Check sheet for the modelled part. Datum: model origin and axes. Units: mm. A direction names the side the tool comes from. Coordinates: 2 decimals unless noted, no trailing zeros. Loops run counter-clockwise (first coordinate to the right, second up) from the corner with the lowest first, then second, coordinate; pieces in that order, holes last. Notation, with made-up numbers: M -17,52.25 L 14,52.25 A19 ccw 14,58.25 Z; hole C -30,9 d7. An arc over 180 degrees is marked long. Answer as CSV lines item,"result". Start each with the question number.
from build123d import *

# Parameters (mm, degrees)
SKETCH052_W     = 15
SKETCH052_H     = 44
PAD029_DEPTH    = 1
SKETCH053_W     = 10.5
SKETCH053_H     = 39.5
PAD030_DEPTH    = 30.5
CHAMFER028_SIZE = 0.5
CHAMFER029_SIZE = 0.5


with BuildPart() as part:
    # Sketch052 → Pad029 (new body)
    with BuildSketch(Plane.XY):
        Rectangle(SKETCH052_W, SKETCH052_H)
    extrude(amount=-PAD029_DEPTH)

    # Sketch053 (on Face5 of Pad029) → Pad030 (join)
    with BuildSketch(Plane.XY):
        Rectangle(SKETCH053_W, SKETCH053_H)
    extrude(amount=PAD030_DEPTH)

    # Chamfer028
    chamfer028_edges = [part.edges().sort_by_distance(p)[0] for p in [
        (-5.25, -19.75, 15.25),
        (5.25, -19.75, 15.25),
        (0, -19.75, 30.5),
        (-5.25, 0, 30.5),
        (5.25, 0, 30.5),
        (5.25, 19.75, 15.25),
        (0, 19.75, 30.5),
        (-5.25, 19.75, 15.25),
    ]]
    chamfer(chamfer028_edges, length=CHAMFER028_SIZE)

    # Chamfer029
    chamfer029_edges = [part.edges().sort_by_distance(p)[0] for p in [
        (0, 22, -1),
        (7.5, 0, -1),
        (0, -22, -1),
        (-7.5, 0, -1),
        (-7.5, -22, -0.5),
        (7.5, -22, -0.5),
        (7.5, 22, -0.5),
        (-7.5, 22, -0.5),
    ]]
    chamfer(chamfer029_edges, length=CHAMFER029_SIZE)


with BuildPart() as part_1:
    # Body010 placement: moved
    add(part.part.moved(Location((-65, 75, -126))))


solid = part_1.part
Item 1: Sectioned sample at C-C, the plane y = 89. Record the boundary of the cut face in (x, z), and give its area (3 significant figures).
Item 2: Sectioned sample at A-A, the plane z = -118.5. Record the boundary of the cut face in (x, y).
Item 3: Go/stop test with flat-tipped pins: pin 1 (9 mm diameter, centred on y = 80.5, z = -109.5, fed in from +X); pin 2 (8 mm diameter, centred on x = -61, z = -113.5, fed in from -Y); pin 3 (15 mm diameter, centred on y = 78, z = -105, fed in from -X). Record where each tip stops, or that it passes through.
Item 4: Sectioned sample at B-B, the plane x = -64.75. Record the boundary of the cut face in (y, z).
Item 5: Material ranges on line 1 (X direction, y = 76, z = -102.5); line 2 (Y direction, x = -68, z = -101); line 3 (Z direction, x = -71.25, y = 77), recorded low to high. Write a range as from..to.
Item 6: Set-up check for faces 1 (the face through (-65, 55.25, -111)), 2 (the face through (-65, 94.75, -111)), 3 (the face through (-70.25, 75, -111)): record each of +Z, -Z, +X, -X, +Y, -Y from which the full face is reachable in a straight line by a thin tool's end or side.
Reply:
1,outline,"M -72.5,-126.5 L -72,-127 L -58,-127 L -57.5,-126.5 L -57.5,-126 L -59.75,-126 L -59.75,-96 L -60.25,-95.5 L -69.75,-95.5 L -70.25,-96 L -70.25,-126 L -72.5,-126 Z"
1,area,"335 mm²"
2,outline,"M -70.25,55.75 L -69.75,55.25 L -60.25,55.25 L -59.75,55.75 L -59.75,94.25 L -60.25,94.75 L -69.75,94.75 L -70.25,94.25 Z"
3,pin 1,"x = -59.75"
3,pin 2,"y = 55.25"
3,pin 3,"x = -70.25"
4,outline,"M 53,-126.5 L 53.5,-127 L 96.5,-127 L 97,-126.5 L 97,-126 L 94.75,-126 L 94.75,-96 L 94.25,-95.5 L 55.75,-95.5 L 55.25,-96 L 55.25,-126 L 53,-126 Z"
5,line 1,"-70.25..-59.75"
5,line 2,"55.25..94.75"
5,line 3,"-127..-126"
6,face 1,"+Z, +X, -X, -Y"
6,face 2,"+Z, +X, -X, +Y"
6,face 3,"+Z, -X, +Y, -Y"
